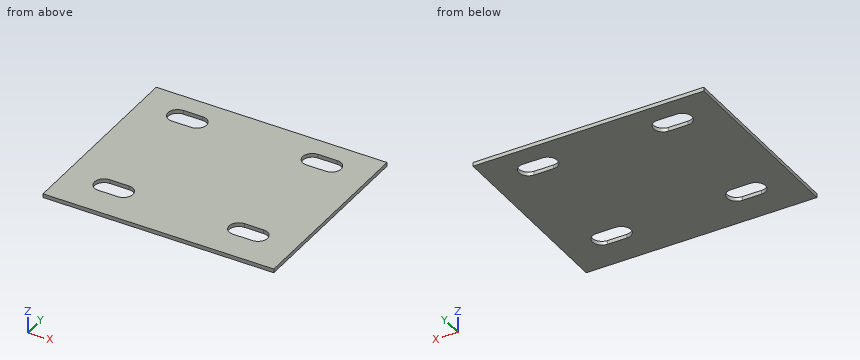
Autodesk Inventor part; units mm, degrees
ref_plane "YZ Plane" through (0, 0, 0) normal (1, 0, 0) x (0, 1, 0)
ref_plane "XZ Plane" through (0, 0, 0) normal (0, 1, 0) x (-1, 0, 0)
ref_plane "XY Plane" through (0, 0, 0) normal (0, 0, 1) x (1, 0, 0)
sketch "Sketch1" plane through (0, 0, 0) normal (0, 0, 1) x (1, 0, 0)
  line L0 (-60, -50) -> (60, -50)
  line L1 (60, -50) -> (60, 50)
  line L2 (60, 50) -> (-60, 50)
  line L3 (-60, 50) -> (-60, -50)
  line L4 (-60, -50) -> (60, 50) construction
  line L5 (60, -50) -> (-60, 50) construction
  line L6 (-60, 0) -> (60, 0) construction
  line L7 (23.5369, 32.6987) -> (33.5369, 32.6987) construction
  line L8 (23.5369, 27.6987) -> (33.5369, 27.6987)
  line L9 (33.5369, 37.6987) -> (23.5369, 37.6987)
  arc A0 (23.5369, 37.6987) -> (23.5369, 27.6987) centre (23.5369, 32.6987) ccw
  arc A1 (33.5369, 27.6987) -> (33.5369, 37.6987) centre (33.5369, 32.6987) ccw
  point P0 (0, 0)
  point P1 (0, 0)
  point P2 (60, 26.1659)
  point P3 (-14.7466, -50)
  point P4 (28.5369, 32.6987)
  dimension "d0" = 120
  dimension "d1" = 100
  dimension "d17" = 5
  dimension "d18" = 10
extrude "Plate1" add sketch "Sketch1" along normal blind 2 contours L3 L2 L1 L0 | A0 L9 A1 L8
sketch "Sketch2" plane through (0, 0, 0) normal (0, 0, -1) x (-1, 0, 0)
  line L0 (-40, 30) -> (160, 30) construction
  line L1 (160, 30) -> (160, 10) construction
  line L2 (160, 10) -> (-40, 10) construction
  line L3 (-40, 10) -> (-40, 30) construction
  line L4 (-60, 50) -> (60, 50)
  line L5 (-60, -50) -> (-60, 50)
  point P0 (0, 0)
  point P1 (-48, 100)
  point P2 (-50, 98)
  point P3 (40, 70)
  point P4 (-60, 26.6315)
  dimension "d6" = 200
  dimension "d9" = 20
  dimension "d10" = 20
  dimension "d11" = 20
mark "Mark1"
sketch "Sketch3" plane through (0, 0, 2) normal (0, 0, 1) x (1, 0, 0)
  line L0 (60, -50) -> (-60, -50)
  line L1 (60, 50) -> (60, -50)
  line L2 (-60, 50) -> (60, 50)
  line L3 (-60, -50) -> (-60, 50)
  line L4 (30, 35) -> (40, 35) construction
  line L5 (30, 30) -> (40, 30)
  line L6 (40, 40) -> (30, 40)
  arc A0 (30, 40) -> (30, 30) centre (30, 35) ccw
  arc A1 (40, 30) -> (40, 40) centre (40, 35) ccw
  point P0 (0, 0)
  point P1 (35, 35)
  dimension "d19" = 5
  dimension "d20" = 10
  dimension "d21" = 15
  dimension "d22" = 25
extrude "Cut1" cut sketch "Sketch3" against normal blind 2 contours A0 L6 A1 L5
pattern_linear "Rectangular Pattern1" count 2 spacing 65 along (0, -1, 0) count 2 spacing 70 along (-1, 0, 0) of "Cut1"
equation "\"d23\" = Thickness"
equation "\"d2\" = Thickness"
equation "\"BendReliefWidth\" = Thickness"
equation "\"BendReliefDepth\" = 0.5 * Thickness"
equation "\"CornerReliefSize\" = 4 * Thickness"
equation "\"MinimumRemnant\" = 2 * Thickness"
equation "\"TransitionRadius\" = BendRadius"
equation "\"JacobiRadiusSize\" = BendRadius"
equation "\"GapSize\" = Thickness"
properties part number "TRM 035 motor pillar 2" material "AISI 304"
Geometry check sheet. Reference: the model listing, model coordinates, mm. Round coordinates to 2 decimals unless told otherwise and drop trailing zeros. Order: outer loops, then holes, each group sorted by start corner. A loop starts at its lowest first (then second) coordinate and runs counter-clockwise, first axis right, second up. Notation, with made-up numbers: (-32.5, 68) -> (6.5, 68) arc R33 cw to (6.5, 105) -> close; hole circle Ø1 at (-22, 25). An arc over 180 degrees is marked (long way). Use one line per item in the form item = value.
1. Cross-section at C-C, the plane z = 0.8. Enter the section's corners in (x, y).
Working result:
outline = (-60, -50) -> (60, -50) -> (60, 50) -> (-60, 50) -> close; hole (-40, -35) -> (-30, -35) arc R5 ccw to (-30, -25) -> (-40, -25) arc R5 ccw to start; hole (-40, 30) -> (-30, 30) arc R5 ccw to (-30, 40) -> (-40, 40) arc R5 ccw to start; hole (30, -35) -> (40, -35) arc R5 ccw to (40, -25) -> (30, -25) arc R5 ccw to start; hole (30, 30) -> (40, 30) arc R5 ccw to (40, 40) -> (30, 40) arc R5 ccw to start
2. Cross-section at B-B, the plane y = -30. Enter the section's corners in (x, z).
Working result:
outline = (-60, 0) -> (-45, 0) -> (-45, 2) -> (-60, 2) -> close; (-25, 0) -> (25, 0) -> (25, 2) -> (-25, 2) -> close; (45, 0) -> (60, 0) -> (60, 2) -> (45, 2) -> close
3. Scan lines: line 1 along X through (y, z) = (-32.5, 0.95); line 2 along X through (y, z) = (37, 0.9); line 3 along Y through (x, z) = (-43.5, 0.3). Record each from-to range of solid material in increasing order. Write a range as from..to.
Working result:
line_1 = -60..-44.33, -25.67..25.67, 44.33..60
line_2 = -60..-44.58, -25.42..25.42, 44.58..60
line_3 = -50..-33.57, -26.43..31.43, 38.57..50
4. Cross-section at A-A, the plane x = 35. Enter the section's corners in (y, z).
Working result:
outline = (-50, 0) -> (-35, 0) -> (-35, 2) -> (-50, 2) -> close; (-25, 0) -> (30, 0) -> (30, 2) -> (-25, 2) -> close; (40, 0) -> (50, 0) -> (50, 2) -> (40, 2) -> close
5. Go/stop test with a flat-tipped pin: pin 1 (1 mm diameter, centred on x = -5.5, y = -28.5, fed in from -Z). Record where the tip stops, or that it passes through.
Working result:
pin_1 = 0
